Autodesk Inventor part; units mm, degrees
ref_plane "YZ Plane" through (0, 0, 0) normal (1, 0, 0) x (0, 1, 0)
ref_plane "XZ Plane" through (0, 0, 0) normal (0, 1, 0) x (-1, 0, 0)
ref_plane "XY Plane" through (0, 0, 0) normal (0, 0, 1) x (1, 0, 0)
sketch "Sketch1" plane through (0, 0, 0) normal (0, 0, 1) x (1, 0, 0)
  line L0 (0, 0) -> (76.2, 0)
  line L1 (76.2, 0) -> (76.2, 73.025)
  line L2 (76.2, 73.025) -> (25.4, 73.025)
  line L3 (0, 50.8) -> (0, 0)
  circle A0 centre (12.7, 38.1) radius 2.0701
  circle A1 centre (12.7, 12.7) radius 2.0701
  line L4 (12.7, 38.1) -> (12.7, 12.7) construction
  line L5 (0, 50.8) -> (25.4, 50.8)
  line L6 (25.4, 50.8) -> (25.4, 73.025)
  dimension "d2" = 4.1402
  dimension "d3" = 4.1402
  dimension "d4" = 12.7
  dimension "d5" = 12.7
  dimension "d6" = 25.4
  dimension "d9" = 25.4
  dimension "d10" = 50.8
  dimension "d11" = 50.8
  dimension "d12" = 73.025
extrude "Extrusion1" add sketch "Sketch1" along normal blind 3.175
properties part number "Polycarbonate Board Circuit Breaker" material "Polycarbonate, Clear"
Work out the finished part from the listing and answer in its coordinate system (mm). A direction names the side the tool comes from. Give positions to 0.01 mm unless a question says otherwise; leave off trailing zeros. Loops run counter-clockwise (first coordinate to the right, second up) from the corner with the lowest first, then second, coordinate; pieces in that order, holes last. Notation, with made-up numbers: (20, -13.75) -> (31, -13.75) arc R20 ccw to (31, 16.25) -> close; hole circle Ø7 at (65, 12.5). An arc over 180 degrees is marked (long way). Put each result on its own line as item: value. Start each with the question number.
Item 1: The part is cut by section A-A (x = 12.7). Give the vertices of the cut face in (y, z) (3 decimals).
Item 2: Each of these flat-tipped pins is pushed along its axis until it touches: P1, Ø3.5, axis at x = 12.7, y = 12.7, coming from the +Z side; P2, Ø3, axis at x = 36.5, y = 26, coming from the -Z side; P3, Ø1, axis at x = 8, z = 2, coming from the +Y side. Where does it stop, or does it pass through?
Item 3: The mould has two halves that part along X. Classify faces 1 (the face through (12.431, 36.048, 1.565)), 2 (the face through (12.431, 10.648, 1.565)), 3 (the face through (0, 26, 2)), 4 (the face through (51, 73.025, 2)): released by +X, released by -X, zero draft, split by the parting line, or undercut.
Item 4: The part is cut by section D-D (y = 61.5). Give the vertices of the cut face in (x, z) (3 decimals), then the cut area to 3 significant figures.
Item 5: The part is cut by section B-B (y = 12.7). Give the vertices of the cut face in (x, z) (3 decimals).
Item 6: The part is cut by section C-C (z = 1.4). Give the vertices of the cut face in (x, y) (3 decimals), then the cut area to 3 significant figures.
Item 7: Which of the six approach directions +Z, -Z, +X, -X, +Y, -Y give full straight-line access (tool end or side, diameter ignored) to faces 5 (the face through (38, 37, 0)), 6 (the face through (25.4, 62, 2))?
Item 8: Find the intervals of material crossed by L1, parallel to Y at x = 12.7, z = 2.1; L2, parallel to X at y = 13, z = 1.65; L3, parallel to Y at x = 11, z = 1.85, in increasing order. Write a range as [from, to].
Answers below:
1. outline: (0, 0) -> (10.63, 0) -> (10.63, 3.175) -> (0, 3.175) -> close; (14.77, 0) -> (36.03, 0) -> (36.03, 3.175) -> (14.77, 3.175) -> close; (40.17, 0) -> (50.8, 0) -> (50.8, 3.175) -> (40.17, 3.175) -> close
2. P1: through
2. P2: z = 0
2. P3: y = 50.8
3. face 1: undercut
3. face 2: undercut
3. face 3: released by -X
3. face 4: zero draft
4. outline: (25.4, 0) -> (76.2, 0) -> (76.2, 3.175) -> (25.4, 3.175) -> close
4. area: 161 mm2
5. outline: (0, 0) -> (10.63, 0) -> (10.63, 3.175) -> (0, 3.175) -> close; (14.77, 0) -> (76.2, 0) -> (76.2, 3.175) -> (14.77, 3.175) -> close
6. outline: (0, 0) -> (76.2, 0) -> (76.2, 73.025) -> (25.4, 73.025) -> (25.4, 50.8) -> (0, 50.8) -> close; hole circle Ø4.14 at (12.7, 12.7); hole circle Ø4.14 at (12.7, 38.1)
6. area: 4,970 mm2
7. face 5: -Z, +X, -X, +Y, -Y
7. face 6: +Z, -Z, -X, +Y
8. L1: [0, 10.63], [14.77, 36.03], [40.17, 50.8]
8. L2: [0, 10.65], [14.75, 76.2]
8. L3: [0, 11.52], [13.88, 36.92], [39.28, 50.8]
